Verification items for this drawing (mm, ordinates from the low corner). A direction names the side the tool comes from. Give positions to 0.01 mm unless a question says otherwise; leave off trailing zeros. Order: outer loops, then holes, each group sorted by start corner. A loop starts at its lowest first (then second) coordinate and runs counter-clockwise, first axis right, second up.
(1) Sectioned sample at A-A on x = 19. Record the cut outline in (y, z), plus the area to 3 significant figures.
(2) Sectioned sample at D-D on x = 35. Record the cut outline in (y, z), plus the area to 3 significant figures.
(3) Scan lines: L1, parallel to X at y = 18, z = 138; L2, parallel to X at y = 33.5, z = 66.5. Record each from-to range of solid material in increasing order.
(4) Gauge pin test, flat end, axial feed: pin 1 (14.5 mm diameter, centred on y = 14, z = 82, fed in from -X). Record the tip position at first contact, or that the pin passes through.
(5) Mould release check, pull along Y, two halves, no side actions. Record for the marked faces 3, 4 and 5: pulls with the +Y half, pulls with the -Y half, needs draft (parallel to the pull), parting line crosses it, or undercut.
(6) Sectioned sample at C-C on z = 36. Record the cut outline in (x, y).
(7) Access from +Z, -Z, +X, -X, +Y, -Y to the whole of each face (thin tool, end or side, straight path). Record for the marked faces 1 and 2.
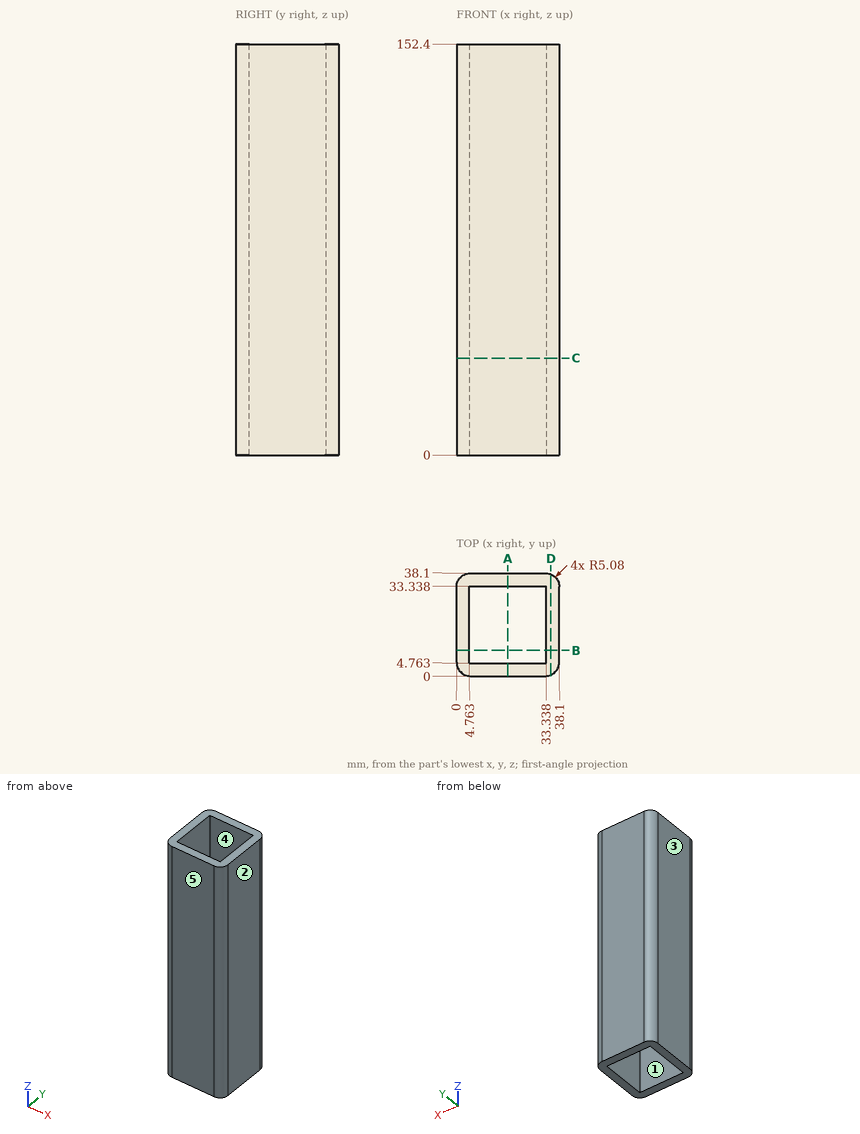
Ans:
1. outline: (0, 0) - (4.76, 0) - (4.76, 152.4) - (0, 152.4) - close; (33.34, 0) - (38.1, 0) - (38.1, 152.4) - (33.34, 152.4) - close
1. area: 1,450 mm2
2. outline: (0.4, 0) - (37.7, 0) - (37.7, 152.4) - (0.4, 152.4) - close
2. area: 5,680 mm2
3. L1: x = 0 to 4.76, 33.34 to 38.1
3. L2: x = 0.02 to 38.08
4. pin 1: stops at x = 0
5. face 3: needs draft
5. face 4: undercut
5. face 5: pulls with the -Y half
6. outline: (0, 5.08) arc R5.08 ccw to (5.08, 0) - (33.02, 0) arc R5.08 ccw to (38.1, 5.08) - (38.1, 33.02) arc R5.08 ccw to (33.02, 38.1) - (5.08, 38.1) arc R5.08 ccw to (0, 33.02) - close; hole (4.76, 4.76) - (33.34, 4.76) - (33.34, 33.34) - (4.76, 33.34) - close
7. face 1: +Z, -Z
7. face 2: +Z, -Z, +X, +Y, -Y
